For this review, take the finished solid that the model builds, in its own axes (mm). A direction names the side the tool comes from. Give positions to 0.01 mm unless a question says otherwise; leave off trailing zeros. Loops run counter-clockwise (first coordinate to the right, second up) from the corner with the lowest first, then second, coordinate; pieces in that order, holes last. Notation, with made-up numbers: (-35.75, 89.5) - (-19.75, 89.5) arc R19 ccw to (-19.75, 112.5) - close; hole circle Ø1 at (7, -0.75). An arc over 180 degrees is marked (long way). Answer as CSV lines item,"result".
from build123d import *

# Parameters (mm, degrees)
BOSS_EXTRUDE1_DEPTH = 14
CHAMFER1_SIZE       = 0.5
CHAMFER2_SIZE       = 0.5
CHAMFER3_SIZE       = 0.5
CHAMFER4_SIZE       = 0.5
CHAMFER5_SIZE       = 0.5
CHAMFER6_SIZE       = 0.5
SKETCH2_R           = 5
CUT_EXTRUDE2_DEPTH  = 14
CUT_EXTRUDE3_DEPTH  = 14
SKETCH4_R           = 2
CUT_EXTRUDE4_DEPTH  = 25
SKETCH5_R           = 2.5
CUT_EXTRUDE5_DEPTH  = 25
CHAMFER7_SIZE       = 0.5
CHAMFER8_SIZE       = 0.5
CHAMFER9_SIZE       = 0.5
CHAMFER10_SIZE      = 0.5
CHAMFER11_SIZE      = 0.5
CHAMFER12_SIZE      = 0.5
CHAMFER13_SIZE      = 0.5
CHAMFER14_SIZE      = 0.5
CHAMFER15_SIZE      = 0.5
CHAMFER16_SIZE      = 0.25
CHAMFER17_SIZE      = 0.25
CHAMFER18_SIZE      = 0.25


with BuildPart() as part:
    # Sketch1 → Boss-Extrude1 (new body)
    with BuildSketch(Plane.XY):
        Polygon((-0.421052632, -3.746003341), (-0.421052632, 23.053996659), (17.578947368, 23.053996659), (17.578947368, -3.746003341), (29.578947368, -3.746003341), (29.578947368, -9.746003341), (-12.421052632, -9.746003341), (-12.421052632, -3.746003341), align=None)
    extrude(amount=BOSS_EXTRUDE1_DEPTH)

    # Chamfer1
    chamfer1_edges = [part.edges().sort_by_distance(p)[0] for p in [
        (17.578947368, -3.746003341, 7),
    ]]
    chamfer(chamfer1_edges, length=CHAMFER1_SIZE)

    # Chamfer2
    chamfer2_edges = [part.edges().sort_by_distance(p)[0] for p in [
        (-0.421052632, -3.746003341, 7),
    ]]
    chamfer(chamfer2_edges, length=CHAMFER2_SIZE)

    # Chamfer3
    chamfer3_edges = [part.edges().sort_by_distance(p)[0] for p in [
        (-12.421052632, -3.746003341, 7),
    ]]
    chamfer(chamfer3_edges, length=CHAMFER3_SIZE)

    # Chamfer4
    chamfer4_edges = [part.edges().sort_by_distance(p)[0] for p in [
        (29.578947368, -3.746003341, 7),
    ]]
    chamfer(chamfer4_edges, length=CHAMFER4_SIZE)

    # Chamfer5
    chamfer5_edges = [part.edges().sort_by_distance(p)[0] for p in [
        (17.578947368, 23.053996659, 7),
    ]]
    chamfer(chamfer5_edges, length=CHAMFER5_SIZE)

    # Chamfer6
    chamfer6_edges = [part.edges().sort_by_distance(p)[0] for p in [
        (-0.421052632, 23.053996659, 7),
    ]]
    chamfer(chamfer6_edges, length=CHAMFER6_SIZE)

    # Sketch2 → Cut-Extrude2 (cut)
    with BuildSketch(Plane.XY.offset(14)):
        with Locations((8.578947368, 10.253996659)):
            Circle(SKETCH2_R)
    extrude(amount=-CUT_EXTRUDE2_DEPTH, mode=Mode.SUBTRACT)

    # Sketch3 → Cut-Extrude3 (cut)
    with BuildSketch(Plane.XY.offset(14)):
        Polygon((8.288550375, 23.332002233), (8.288550375, 14.543053955), (8.869344362, 14.973079178), (8.869344362, 23.332002233), align=None)
    extrude(amount=-CUT_EXTRUDE3_DEPTH, mode=Mode.SUBTRACT)

    # Sketch4 → Cut-Extrude4 (cut)
    with BuildSketch(Plane(origin=(17.578947368, 0, 0), x_dir=(0, 0, -1), z_dir=(1, 0, 0))):
        with Locations((-7, 19.481136132)):
            Circle(SKETCH4_R)
    extrude(amount=-CUT_EXTRUDE4_DEPTH, mode=Mode.SUBTRACT)

    # Sketch5 → Cut-Extrude5 (cut)
    with BuildSketch(Plane.XZ.offset(9.746003341)):
        with Locations((-7.421052632, 7)):
            Circle(SKETCH5_R)
        with Locations((24.578947368, 7)):
            Circle(SKETCH5_R)
    extrude(amount=-CUT_EXTRUDE5_DEPTH, mode=Mode.SUBTRACT)

    # Chamfer7
    chamfer7_edges = [part.edges().sort_by_distance(p)[0] for p in [
        (-9.921052632, -3.746003341, 7),
    ]]
    chamfer(chamfer7_edges, length=CHAMFER7_SIZE)

    # Chamfer8
    chamfer8_edges = [part.edges().sort_by_distance(p)[0] for p in [
        (22.078947368, -3.746003341, 7),
    ]]
    chamfer(chamfer8_edges, length=CHAMFER8_SIZE)

    # Chamfer9
    chamfer9_edges = [part.edges().sort_by_distance(p)[0] for p in [
        (23.578947368, -3.746003341, 14),
    ]]
    chamfer(chamfer9_edges, length=CHAMFER9_SIZE)

    # Chamfer10
    chamfer10_edges = [part.edges().sort_by_distance(p)[0] for p in [
        (18.328947368, -3.996003341, 14),
    ]]
    chamfer(chamfer10_edges, length=CHAMFER10_SIZE)

    # Chamfer11
    chamfer11_edges = [part.edges().sort_by_distance(p)[0] for p in [
        (23.578947368, -3.746003341, 0),
    ]]
    chamfer(chamfer11_edges, length=CHAMFER11_SIZE)

    # Chamfer12
    chamfer12_edges = [part.edges().sort_by_distance(p)[0] for p in [
        (18.328947368, -3.996003341, 0),
    ]]
    chamfer(chamfer12_edges, length=CHAMFER12_SIZE)

    # Chamfer13
    chamfer13_edges = [part.edges().sort_by_distance(p)[0] for p in [
        (4.183748872, 23.053996659, 0),
        (12.974145865, 23.053996659, 0),
    ]]
    chamfer(chamfer13_edges, length=CHAMFER13_SIZE)

    # Chamfer14
    chamfer14_edges = [part.edges().sort_by_distance(p)[0] for p in [
        (12.974145865, 23.053996659, 14),
        (4.183748872, 23.053996659, 14),
    ]]
    chamfer(chamfer14_edges, length=CHAMFER14_SIZE)

    # Chamfer15
    chamfer15_edges = [part.edges().sort_by_distance(p)[0] for p in [
        (-0.671052632, -3.496003341, 0),
        (-6.421052632, -3.746003341, 0),
        (-0.671052632, -3.496003341, 14),
        (-6.421052632, -3.746003341, 14),
    ]]
    chamfer(chamfer15_edges, length=CHAMFER15_SIZE)

    # Chamfer16
    chamfer16_edges = [part.edges().sort_by_distance(p)[0] for p in [
        (5.147619999, 6.617240896, 0),
        (5.147619999, 6.617240896, 14),
    ]]
    chamfer(chamfer16_edges, length=CHAMFER16_SIZE)

    # Chamfer17
    chamfer17_edges = [part.edges().sort_by_distance(p)[0] for p in [
        (-0.421052632, 19.481136132, 9),
    ]]
    chamfer(chamfer17_edges, length=CHAMFER17_SIZE)

    # Chamfer18
    chamfer18_edges = [part.edges().sort_by_distance(p)[0] for p in [
        (17.578947368, 19.481136132, 9),
    ]]
    chamfer(chamfer18_edges, length=CHAMFER18_SIZE)


solid = part.part
1) Consider section D-D on x = 21. Write out the cut boundary in (y, z).
From the geometry:
outline,"(-9.75, 0) - (-4.25, 0) - (-3.75, 0.5) - (-3.75, 13.5) - (-4.25, 14) - (-9.75, 14) - close"
2) Wall thickness on line 1 (X direction, y = 21.5, z = 5.5); line 2 (Y direction, x = -9.5, z = 10); line 3 (X direction, y = -0.5, z = 0.5): over which ranges is each line inside the solid? List them lowest first. Write a range as from..to.
From the geometry:
line 1,"x = -0.42..8.29, 8.87..17.58"
line 2,"y = -9.75..-3.75"
line 3,"x = -0.42..17.58"
3) Consider section C-C on z = 12. Write out the cut boundary in (x, y), and give its area (3 significant figures).
From the geometry:
outline,"(-12.42, -9.75) - (29.58, -9.75) - (29.58, -4.25) - (29.08, -3.75) - (18.08, -3.75) - (17.58, -3.25) - (17.58, 22.55) - (17.08, 23.05) - (8.87, 23.05) - (8.87, 15.25) arc R5 cw (long way) to (8.29, 15.25) - (8.29, 23.05) - (0.08, 23.05) - (-0.42, 22.55) - (-0.42, -3.25) - (-0.92, -3.75) - (-11.92, -3.75) - (-12.42, -4.25) - close"
area,"651 mm^2"
4) Machinability: for faces 1 (the flat face through (9, 2, 14)), 2 (the cylindrical face through (-5.112, -7.035, 6.042)), 3 (the flat face through (-4, -3.746, 7)), 4 (the flat face through (21, -3.746, 7)), 5 (the flat face through (8.869, 17, 7)), which of the approach directions +Z, -Z, +X, -X, +Y, -Y give a long, thin tool a straight path to every point of the face, cutting with its end or side? Answer none if there is none.
From the geometry:
face 1,"+Z, +X, -X, +Y, -Y"
face 2,"+Y, -Y"
face 3,"+Z, -Z, -X, +Y"
face 4,"+Z, -Z, +X, +Y"
face 5,"+Z, -Z, +Y"
5) Consider section A-A on y = -6. Write out the cut boundary in (x, z).
From the geometry:
outline,"(-12.42, 0) - (29.58, 0) - (29.58, 14) - (-12.42, 14) - close; hole circle Ø5 at (-7.42, 7); hole circle Ø5 at (24.58, 7)"
6) Draft analysis for pull direction Y (two halves, no side actions). For faces 6 (the flat face through (4, 23.054, 7)), 7 (the flat face through (9, 2, 0)), 8 (the cylindrical face through (13.158, 20.833, 8.474)), state which applies: pulls with the +Y half, pulls with the -Y half, needs draft (parallel to the pull), parting line crosses it, or undercut.
From the geometry:
face 6,"pulls with the +Y half"
face 7,"needs draft"
face 8,"undercut"
7) Consider section B-B on z = 7. Count the separate pieces of the cut face and the enclosed holes in it, and give its area (3 significant figures).
From the geometry:
separate pieces,"5"
enclosed holes,"0"
area,"521 mm^2"
8) Insertion check: P1, Ø7, axis at y = 6, z = 8.5, coming from the +X side; P2, Ø3, axis at y = 16, z = 2, coming from the -X side; P3, Ø8, axis at x = -7.42, z = 7, coming from the +Y side. Each pin has a flat end and moves straight along its axis. Give the tip position at first contact, or say it passes through.
From the geometry:
P1,"stops at x = 17.58"
P2,"stops at x = -0.42"
P3,"stops at y = -3.75"
